from build123d import *

# Parameters (mm, degrees)
BOX010_W     = 6.2
BOX010_H     = 6.1
BOX010_DEPTH = 50
BOX009_W     = 6.2
BOX009_H     = 6.1
BOX009_DEPTH = 50
BOX007_W     = 6.1
BOX007_H     = 6.2
BOX007_DEPTH = 50
BOX006_W     = 6.1
BOX006_H     = 6.2
BOX006_DEPTH = 50
BOX005_W     = 11
BOX005_H     = 1.6
BOX005_DEPTH = 50
BOX004_W     = 11
BOX004_H     = 1.6
BOX004_DEPTH = 50
BOX002_W     = 1.6
BOX002_H     = 11
BOX002_DEPTH = 50
BOX001_W     = 1.6
BOX001_H     = 11
BOX001_DEPTH = 52
BOX_W        = 20
BOX_H        = 20
BOX_DEPTH    = 40


with BuildPart() as cube009:
    # Box010 → Box010 (new body)
    with BuildSketch(Plane(origin=(6.9, 13.9, -7), x_dir=(1, 0, 0), z_dir=(0, 0, 1))):
        with Locations((3.1, 3.05)):
            Rectangle(BOX010_W, BOX010_H)
    extrude(amount=BOX010_DEPTH)


with BuildPart() as cube008:
    # Box009 → Box009 (new body)
    with BuildSketch(Plane(origin=(6.9, 0, -7), x_dir=(1, 0, 0), z_dir=(0, 0, 1))):
        with Locations((3.1, 3.05)):
            Rectangle(BOX009_W, BOX009_H)
    extrude(amount=BOX009_DEPTH)


with BuildPart() as cube006:
    # Box007 → Box007 (new body)
    with BuildSketch(Plane(origin=(13.9, 6.9, -7), x_dir=(1, 0, 0), z_dir=(0, 0, 1))):
        with Locations((3.05, 3.1)):
            Rectangle(BOX007_W, BOX007_H)
    extrude(amount=BOX007_DEPTH)


with BuildPart() as cube005:
    # Box006 → Box006 (new body)
    with BuildSketch(Plane(origin=(0, 6.9, -7), x_dir=(1, 0, 0), z_dir=(0, 0, 1))):
        with Locations((3.05, 3.1)):
            Rectangle(BOX006_W, BOX006_H)
    extrude(amount=BOX006_DEPTH)


with BuildPart() as cube004:
    # Box005 → Box005 (new body)
    with BuildSketch(Plane(origin=(4.5, 16.6, -6), x_dir=(1, 0, 0), z_dir=(0, 0, 1))):
        with Locations((5.5, 0.8)):
            Rectangle(BOX005_W, BOX005_H)
    extrude(amount=BOX005_DEPTH)


with BuildPart() as cube003:
    # Box004 → Box004 (new body)
    with BuildSketch(Plane(origin=(4.5, 1.8, -3), x_dir=(1, 0, 0), z_dir=(0, 0, 1))):
        with Locations((5.5, 0.8)):
            Rectangle(BOX004_W, BOX004_H)
    extrude(amount=BOX004_DEPTH)


with BuildPart() as cube001:
    # Box002 → Box002 (new body)
    with BuildSketch(Plane(origin=(16.6, 4.5, -6), x_dir=(1, 0, 0), z_dir=(0, 0, 1))):
        with Locations((0.8, 5.5)):
            Rectangle(BOX002_W, BOX002_H)
    extrude(amount=BOX002_DEPTH)


with BuildPart() as obj1:
    # Box001 → Box001 (new body)
    with BuildSketch(Plane(origin=(1.8, 4.5, -2), x_dir=(1, 0, 0), z_dir=(0, 0, 1))):
        with Locations((0.8, 5.5)):
            Rectangle(BOX001_W, BOX001_H)
    extrude(amount=BOX001_DEPTH)


with BuildPart() as cut007:
    # Box → Box (new body)
    with BuildSketch(Plane.XY):
        with Locations((10, 10)):
            Rectangle(BOX_W, BOX_H)
    extrude(amount=BOX_DEPTH)

    # Cut: cut obj1
    add(obj1.part, mode=Mode.SUBTRACT)


with BuildPart() as cut007_1:
    # Cut placement: moved
    add(cut007.part.moved(Location((0, 0, -3))))

    # Cut001: cut Cube001
    add(cube001.part, mode=Mode.SUBTRACT)

    # Cut002: cut Cube003
    add(cube003.part, mode=Mode.SUBTRACT)

    # Cut003: cut Cube004
    add(cube004.part, mode=Mode.SUBTRACT)

    # Cut004: cut Cube005
    add(cube005.part, mode=Mode.SUBTRACT)

    # Cut005: cut Cube006
    add(cube006.part, mode=Mode.SUBTRACT)

    # Cut006: cut Cube008
    add(cube008.part, mode=Mode.SUBTRACT)

    # Cut007: cut Cube009
    add(cube009.part, mode=Mode.SUBTRACT)


solid = cut007_1.part
Design review of the part built by this model. Coordinates are the model's own, in mm. A direction names the side the tool comes from. Coordinates: 2 decimals unless noted, no trailing zeros. Loops run counter-clockwise (first coordinate to the right, second up) from the corner with the lowest first, then second, coordinate; pieces in that order, holes last. Notation, with made-up numbers: M 89.5,-35.5 L 104.5,-35.5 A19 cw 104.5,1.5 Z; hole C 32.5,-22 d11. An arc over 180 degrees is marked long. Answer as CSV lines item,"result".
Item 1: Machinability: for faces 4 (the face through (13.9, 10, 17)), 5 (the face through (13.1, 15, 17)), 6 (the face through (6.9, 5, 17)), 7 (the face through (4.5, 3, 17)), 8 (the face through (1, 6.9, 17)), which of the approach directions +Z, -Z, +X, -X, +Y, -Y give a long, thin tool a straight path to every point of the face, cutting with its end or side? Answer none if there is none.
Answer list:
face 4,"+Z, -Z, +X"
face 5,"+Z, -Z, +Y"
face 6,"+Z, -Z, -Y"
face 7,"+Z, -Z"
face 8,"+Z, -Z, -X"
Item 2: Add section C-C on x = 15. State the section outline as (y, z) points.
Answer list:
outline,"M 0,-3 L 1.8,-3 L 1.8,37 L 0,37 Z; M 3.4,-3 L 6.9,-3 L 6.9,37 L 3.4,37 Z; M 13.1,-3 L 16.6,-3 L 16.6,37 L 13.1,37 Z; M 18.2,-3 L 20,-3 L 20,37 L 18.2,37 Z"
Item 3: For P1, Ø8, axis at x = 5.5, z = 4.5, coming from the -Y side, flat-tipped, find the tip position at first contact; note if it passes through.
Answer list:
P1,"y = 0"
Item 4: The part is to be moulded in two halves that separate along Y. For faces 1 (the face through (6.9, 19, 17)), 2 (the face through (14, 1.8, 17)), 3 (the face through (10, 13.9, 17)), say which applies: pulls with the +Y half, pulls with the -Y half, needs draft (parallel to the pull), parting line crosses it, or undercut.
Answer list:
face 1,"needs draft"
face 2,"undercut"
face 3,"pulls with the +Y half"
Item 5: For probe 1 along Y at (x, z) = (5.75, 0.5); probe 2 along Y at (x, z) = (19.25, 34.5), list the stretches that pass through material, from the lowest coordinate up.
Answer list:
probe 1,"0 to 1.8, 3.4 to 6.9, 13.1 to 16.6, 18.2 to 20"
probe 2,"0 to 6.9, 13.1 to 20"
Item 6: Add section A-A on y = 17. State the section outline as (x, z) points, plus the area to 3 significant figures.
Answer list:
outline,"M 0,-3 L 4.5,-3 L 4.5,37 L 0,37 Z; M 15.5,-3 L 20,-3 L 20,37 L 15.5,37 Z"
area,"360 mm²"
Item 7: Add section B-B on x = 4. State the section outline as (y, z) points.
Answer list:
outline,"M 0,-3 L 6.9,-3 L 6.9,37 L 0,37 Z; M 13.1,-3 L 20,-3 L 20,37 L 13.1,37 Z"
